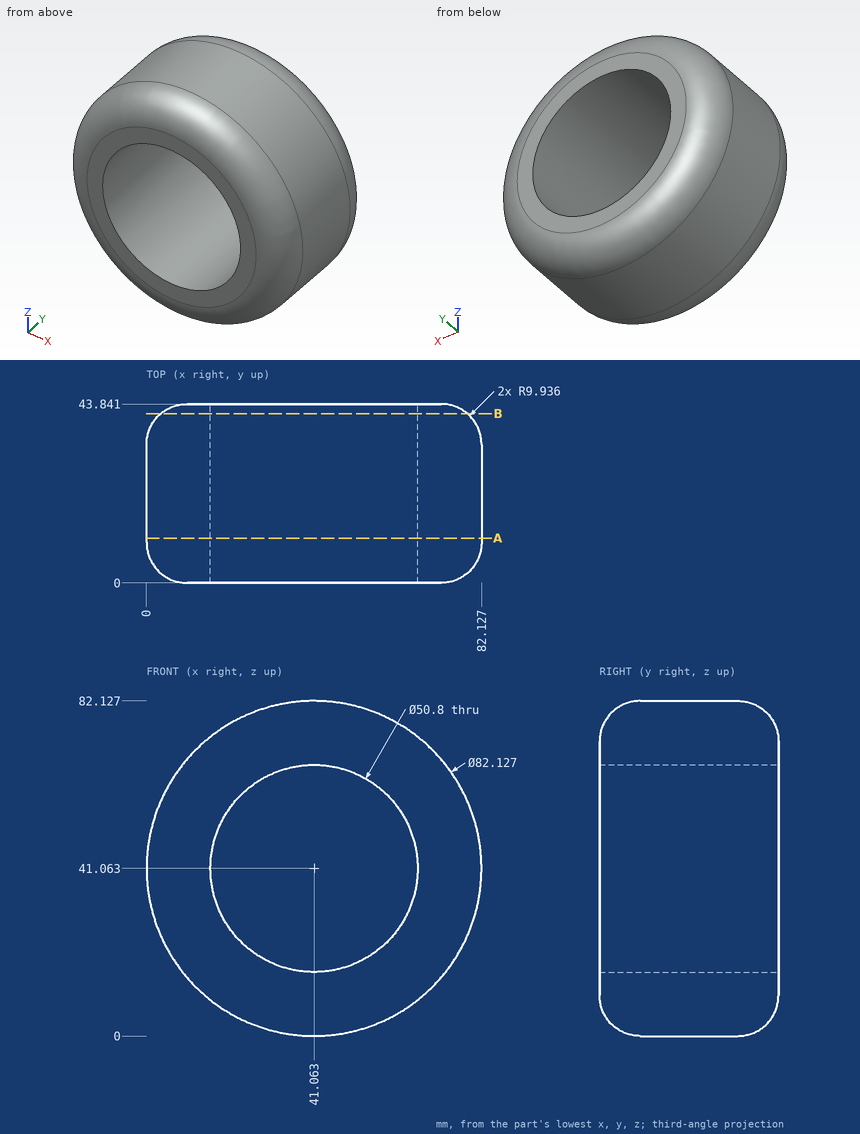
The drawing under review shows one solid part. Ordinate dimensions are in mm from its lowest x, y, z. Give positions to 0.01 mm unless a question says otherwise; leave off trailing zeros. Order: outer loops, then holes, each group sorted by start corner. A loop starts at its lowest first (then second) coordinate and runs counter-clockwise, first axis right, second up. Notation, with made-up numbers: M 21,42.5 L 38,42.5 A20 cw 38,76.5 Z; hole C 68.5,38 d10. An arc over 180 degrees is marked long. Answer in a Markdown table with one row per item. Add a question column.
1. Add section A-A on y = 11. State the section outline as (x, z) points.
2. Add section B-B on y = 41.5. State the section outline as (x, z) points.
3. To check wall thickness, follow line 1 along X through (y, z) = (17, 40.5); line 2 along Z through (x, y) = (29, 29) (1 decimal); line 3 along X through (y, z) = (27.5, 39) (1 decimal). State the ranges of each line that lie inside material, in increasing order.
4. For pin 1 Ø3 at (x, y) = (25, 30) entering from +Z; pin 2 Ø12 at (x, y) = (36.5, 34) entering from +Z; pin 3 Ø5 at (y, z) = (11, 68) entering from -X, all flat-tipped, find the tip position at first contact; note any pin that passes through.
The answers:
| question | item | result |
|---|---|---|
| 1 | outline | C 41.06,41.06 d82.13; hole C 41.06,41.06 d50.8 |
| 2 | outline | C 41.06,41.06 d75.07; hole C 41.06,41.06 d50.8 |
| 3 | line 1 | 0 to 15.67, 66.46 to 82.12 |
| 3 | line 2 | 1.8 to 18.7, 63.4 to 80.3 |
| 3 | line 3 | 0.1 to 15.7, 66.4 to 82.1 |
| 4 | pin 1 | z = 79.46 |
| 4 | pin 2 | z = 82.13 |
| 4 | pin 3 | x = 8.06 |
